```python
from build123d import *

# Parameters (mm, degrees)
F0_R     = 12.5
F0_R_2   = 7.5
F1_DEPTH = 3.4
F2_R     = 3
F4_R     = 1.5
F5_DEPTH = 10


# Not quite as in the source:
# - the program builds the solid bodies; features that only make, move or delete a surface that nothing else refers to are left out


with BuildPart() as f1:
    # F0 (on Front) → F1 (new body, symmetric)
    with BuildSketch(Plane.XZ):
        Circle(F0_R)
        Circle(F0_R_2, mode=Mode.SUBTRACT)
    extrude(amount=F1_DEPTH, both=True)

    # F2
    f2_edges = [f1.edges().sort_by_distance(p)[0] for p in [
        (-12.5, 3.4, 0),
        (-12.5, -3.4, 0),
    ]]
    fillet(f2_edges, radius=F2_R)

    # F4 (on Right) → F5 (join, symmetric)
    with BuildSketch(Plane.YZ):
        Circle(F4_R)
    extrude(amount=F5_DEPTH, both=True)


solid = f1.part
```
The model under review builds one solid part; all positions refer to its coordinate system, in mm. Coordinates: 2 decimals unless noted, no trailing zeros. Write each loop counter-clockwise with the first axis right and the second up, starting at its lowest first coordinate (ties: lowest second). Pieces come first, ordered by that corner, then holes.
1) The part is to be moulded in two halves that separate along X. For faces 1 (the face through (0.11, -1.5, 0.07)), 2 (the face through (1, 3.4, 8)), 3 (the face through (11.923, -0.006, 3.755)), say which applies: pulls with the +X half, pulls with the -X half, needs draft (parallel to the pull), parting line crosses it, or undercut.
2) We need section C-C on y = 0. State the section outline as (x, z) points.
3) We need section B-B on z = 0. State the section outline as (x, y) points, then the cut area to 3 significant figures.
4) To check wall thickness, follow probe 1 along Z at (x, y) = (-3, 0.75); probe 2 along Z at (x, y) = (-5.5, -0.25); probe 3 along Z at (x, y) = (-1, 2.25). State the ranges of each line that lie inside material, in increasing order.
5) We need section D-D on y = 2.5. State the section outline as (x, z) points.
6) We need section A-A on x = 0. State the section outline as (y, z) points.
7) Clearance check with flat-ended pins moving along their axes: pin 1 Ø2 at (x, y) = (-7, 0.5) entering from -Z; pin 2 Ø1.5 at (x, z) = (0, 3) entering from -Y; pin 3 Ø1.5 at (x, z) = (7, 9.5) entering from +Y; pin 4 Ø4 at (x, y) = (3, -2) entering from +Z. State where each tip first meets the part, or that it passes through.
Answer list:
1. face 1: undercut
1. face 2: needs draft
1. face 3: parting line crosses it
2. outline: circle Ø25 at (0, 0); hole (-7.35, -1.5) arc R7.5 ccw to (7.35, -1.5) - close; hole (-7.35, 1.5) - (7.35, 1.5) arc R7.5 ccw to start
3. outline: (-12.5, -0.4) arc R3 ccw to (-9.5, -3.4) - (-7.5, -3.4) - (-7.5, -1.5) - (7.5, -1.5) - (7.5, -3.4) - (9.5, -3.4) arc R3 ccw to (12.5, -0.4) - (12.5, 0.4) arc R3 ccw to (9.5, 3.4) - (7.5, 3.4) - (7.5, 1.5) - (-7.5, 1.5) - (-7.5, 3.4) - (-9.5, 3.4) arc R3 ccw to (-12.5, 0.4) - close
3. area: 105 mm2
4. probe 1: z = -12.11 to -6.87, -1.3 to 1.3, 6.87 to 12.11
4. probe 2: z = -11.22 to -5.1, -1.48 to 1.48, 5.1 to 11.22
4. probe 3: z = -11.82 to -7.43, 7.43 to 11.82
5. outline: circle Ø23.28 at (0, 0); hole circle Ø15 at (0, 0)
6. outline: (-3.4, -9.5) arc R3 ccw to (-0.4, -12.5) - (0.4, -12.5) arc R3 ccw to (3.4, -9.5) - (3.4, -7.5) - (-3.4, -7.5) - close; (-3.4, 7.5) - (3.4, 7.5) - (3.4, 9.5) arc R3 ccw to (0.4, 12.5) - (-0.4, 12.5) arc R3 ccw to (-3.4, 9.5) - close; circle Ø3 at (0, 0)
7. pin 1: stops at z = -10.96
7. pin 2: passes through
7. pin 3: stops at y = 2.97
7. pin 4: stops at z = 12.4
